The model under review builds one solid part; all positions refer to its coordinate system, in mm. Coordinates: 2 decimals unless noted, no trailing zeros. Write each loop counter-clockwise with the first axis right and the second up, starting at its lowest first coordinate (ties: lowest second). Pieces come first, ordered by that corner, then holes. Notation, with made-up numbers: (15.5, 63.25) - (71.5, 63.25) arc R17 cw to (71.5, 93.25) - close; hole circle Ø8 at (-23.75, 71.5). An arc over 180 degrees is marked (long way). Put each result on its own line as item: value.
Autodesk Inventor part; units mm, degrees
ref_plane "IDS_WORKPLANE" through (626.4664, 0, 0) normal (1, 0, 0) x (0, 0, -1)
ref_plane "Work Plane2" through (325, 0, 0) normal (0, 0, -1) x (1, 0, 0)
ref_plane "YZ Plane" through (0, 0, 0) normal (1, 0, 0) x (0, 1, 0)
sketch "Sketch1" plane through (0, 0, 0) normal (0, 0, 1) x (1, 0, 0)
  line L0 (0, 0) -> (0, 12)
  line L1 (0, 12) -> (650, 12)
  line L2 (650, 12) -> (650, 0)
  line L3 (650, 0) -> (0, 0)
  line L4 (0, 14.4) -> (0, -2.4)
  line L5 (-130, 0) -> (780, 0)
  dimension "d0" = 24
  dimension "d1" = 650
revolve "Body" add sketch "Sketch1" angle 360 about axis through (650, 0, 0) along (-1, 0, 0)
chamfer "Chamfer1" distance 1.5346 distance2 1.5336 1 edges at (650, -12, 0) measured on face at (650, -0.5646, -3.2919)
sketch "Sketch2" plane through (0, 0, 0) normal (0, 0, 1) x (1, 0, 0)
  line L0 (0, 1.5) -> (5.2, 1.5)
  line L1 (5.2, 1.5) -> (5.2, -1.5)
  line L2 (5.2, -1.5) -> (0, -1.5)
  line L3 (0, -12) -> (0, 12)
  line L4 (-1.04, 0) -> (6.24, 0)
  dimension "d7" = 1.5
  dimension "d8" = 5.2
extrude "Slot" cut sketch "Sketch2" along normal through all both and the other way through all
chamfer "Chamfer2" distance 2 angle 45 2 edges at (0, 9, 7.9373) (0, 9, -7.9373) measured on face at (0, 4.5446, 1.8536)
chamfer "Chamfer3" distance 2 angle 45 1 edges at (0, -12, 0) measured on face at (0, -7.3845, 2.2772)
ref_plane "IDS_WORKPLANE" through (626.4664, 0, 0) normal (1, 0, 0) x (0, 0, -1)
ref_plane "Work Plane2" through (325, 0, 0) normal (0, 0, -1) x (1, 0, 0)
thread "Thread2"
equation "\"d7\" = 0.5 * SBR"
equation "\"d8\" = STI"
equation "\"d6\" = -0.5 * GD1 + 0.5 * NND"
equation "\"d11\" = 0.1 * NND"
equation "\"d20\" = 0.1 * NND"
equation "\"d13\" = 0.1 * NND"
equation "\"d21\" = 0.1 * NND"
equation "\"GEL\" = 22"
equation "\"SBR\" = 3"
equation "\"STI\" = 5.2"
equation "\"GD1\" = THREADDIA - 1.2269 * PTC"
equation "\"GAL\" = 0.61345 * PTC"
equation "\"GUL\" = 0.61345 * PTC"
equation "\"d16\" = -GAL - GEL"
equation "\"d17\" = -GAL - GEL"
equation "\"TOA\" = 30deg"
equation "\"PTC\" = 2.5"
properties part number "DIN 427 - M20 x 60" material "Steel, Mild"
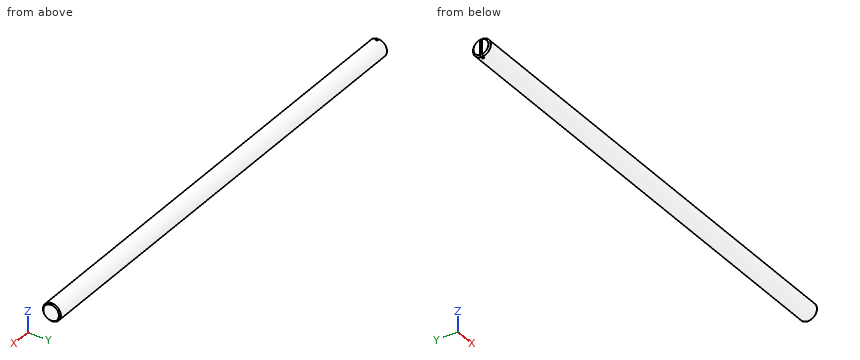
1. For pin 1 Ø12 at (x, z) = (325, -8.5) entering from -Y; pin 2 Ø2.5 at (x, z) = (2.5, -1.5) entering from -Y; pin 3 Ø8 at (x, y) = (190.5, 6.5) entering from +Z, all flat-tipped, find the tip position at first contact; note any pin that passes through.
Determined:
pin 1: stops at y = -11.74
pin 2: stops at y = -12
pin 3: stops at z = 11.74
2. To check wall thickness, follow probe 1 along Y at (x, z) = (406, 2.25); probe 2 along X at (y, z) = (0.25, 9); probe 3 along Y at (x, z) = (609.5, -1). State the ranges of each line that lie inside material, in increasing order.
Determined:
probe 1: y = -11.79 to 11.79
probe 2: x = 5.2 to 650
probe 3: y = -11.96 to 11.96
3. Consider section A-A on x = 461. State the section outline as (y, z) points.
Determined:
outline: circle Ø24 at (0, 0)
